Here's how the part is built. I have some questions about the finished solid (model axes, mm). Face numbers are marked on the shaded views. A direction names the side the tool comes from. Round coordinates to 2 decimals unless told otherwise and drop trailing zeros. Loops run counter-clockwise (first coordinate to the right, second up) from the corner with the lowest first, then second, coordinate; pieces in that order, holes last. Notation, with made-up numbers: (41.25, 33) -> (55.25, 33) arc R3 ccw to (55.25, 37) -> close; hole circle Ø5 at (38.5, 23). An arc over 180 degrees is marked (long way). One line per item, written item: value. Start each with the question number.
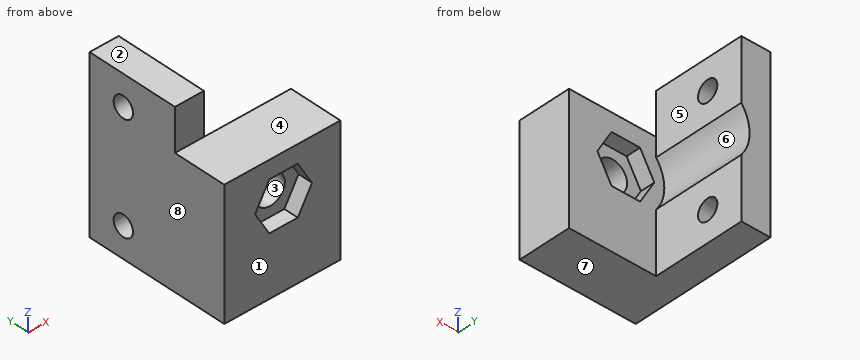
```python
from build123d import *

# Parameters (mm, degrees)
SKETCH1_W           = 18
SKETCH1_H           = 35
SKETCH1_R           = 3.05
BOSS_EXTRUDE1_DEPTH = 11
SKETCH1_3_W         = 6
SKETCH1_3_H         = 35
BOSS_EXTRUDE2_DEPTH = 30
SKETCH2_R           = 7.949273458
CUT_EXTRUDE1_DEPTH  = 19
CUT_EXTRUDE3_DEPTH  = 3
CUT_EXTRUDE4_DEPTH  = 3
SKETCH7_R           = 2.15
CUT_EXTRUDE6_DEPTH  = 10
SKETCH8_W           = 24
SKETCH8_H           = 8.700587772
CUT_EXTRUDE7_DEPTH  = 11


with BuildPart() as part:
    # Sketch1 → Boss-Extrude1 (new body)
    with BuildSketch(Plane(origin=(0, 0, 0), x_dir=(1, 0, 0), z_dir=(0, 1, 0))):
        with Locations((12, 0)):
            Rectangle(SKETCH1_W, SKETCH1_H)
        with Locations((9.25, 0)):
            Circle(SKETCH1_R, mode=Mode.SUBTRACT)
    extrude(amount=BOSS_EXTRUDE1_DEPTH)

    # Sketch1<3> → Boss-Extrude2 (add)
    with BuildSketch(Plane(origin=(0, 0, 0), x_dir=(1, 0, 0), z_dir=(0, 1, 0))):
        Rectangle(SKETCH1_3_W, SKETCH1_3_H)
    extrude(amount=BOSS_EXTRUDE2_DEPTH)

    # Sketch2 → Cut-Extrude1 (cut)
    with BuildSketch(Plane(origin=(0, 30, 0), x_dir=(1, 0, 0), z_dir=(0, 1, 0))):
        with Locations((9.25, 0)):
            Circle(SKETCH2_R)
    extrude(amount=-CUT_EXTRUDE1_DEPTH, mode=Mode.SUBTRACT)

    # Sketch4 → Cut-Extrude3 (cut)
    with BuildSketch(Plane(origin=(0, 11, 0), x_dir=(1, 0, 0), z_dir=(0, 1, 0))):
        Polygon((15.138972746, 0), (12.194486373, 5.1), (6.305513627, 5.1), (3.361027254, 0), (6.305513627, -5.1), (12.194486373, -5.1), align=None)
    extrude(amount=-CUT_EXTRUDE3_DEPTH, mode=Mode.SUBTRACT)

    # Sketch5 → Cut-Extrude4 (cut)
    with BuildSketch(Plane.XZ):
        Polygon((3.361027254, 0), (6.305513627, -5.1), (12.194486373, -5.1), (15.138972746, 0), (12.194486373, 5.1), (6.305513627, 5.1), align=None)
    extrude(amount=-CUT_EXTRUDE4_DEPTH, mode=Mode.SUBTRACT)

    # Sketch7 → Cut-Extrude6 (cut)
    with BuildSketch(Plane(origin=(3, 0, 0), x_dir=(0, 0, -1), z_dir=(1, 0, 0))):
        with Locations((-11.206035856, 22.5)):
            Circle(SKETCH7_R)
        with Locations((11.206035856, 22.5)):
            Circle(SKETCH7_R)
    extrude(amount=-CUT_EXTRUDE6_DEPTH, mode=Mode.SUBTRACT)

    # Sketch8 → Cut-Extrude7 (cut)
    with BuildSketch(Plane.XZ):
        with Locations((9, 13.149706114)):
            Rectangle(SKETCH8_W, SKETCH8_H)
    extrude(amount=-CUT_EXTRUDE7_DEPTH, mode=Mode.SUBTRACT)


solid = part.part
```
Q1. Will these pins go through, and if not, where does the flat tip stop? P1, Ø3.5, axis at y = 22.5, z = -11.21, coming from the +X side; P2, Ø4, axis at y = 17, z = -8, coming from the +X side; P3, Ø2.5, axis at x = 8, y = 2, coming from the +Z side; P4, Ø3, axis at x = 0, z = 12.5, coming from the -Y side.
Q2. I want a section at D-D on z = 6.5. Please give me the cut outline in (x, y), plus the area to 3 significant figures.
Q3. Which directions (+Z, -Z, +X, -X, +Y, -Y) give clear straight access to the entire face, cutting with the end or side of a thin tool? Please do the marked faces 4, 5, 6, 7 and 8.
Q4. I want a section at C-C on y = 22.5. Please give me the cut outline in (x, z), plus the area to 3 significant figures.
Q5. If I drill on line 1 along Z through (x, y) = (9.25, 6.15); line 2 along X through (y, z) = (26, -16); line 3 along Y through (x, z) = (15.75, -12), over which ranges is the centre line in solid material (lowest first)?
Q6. I want a section at B-B on y = 10. Please give me the cut outline in (x, z).
Q7. I want a section at A-A on x = 9.25. Please give me the cut outline in (y, z), plus the area to 3 significant figures.
Q8. If we mould it in two halves opening along Z, with no side actions, what happens to the marked faces 1, 2 and 3? For each: released by +Z, released by -Z, zero draft, split by the parting line, or undercut.
Answers below:
1. P1: passes through
1. P2: stops at x = 3
1. P3: stops at z = 8.8
1. P4: stops at y = 11
2. outline: (-3, 0) -> (21, 0) -> (21, 11) -> (3, 11) -> (3, 30) -> (-3, 30) -> close
2. area: 378 mm^2
3. face 4: +Z, +X, -X, -Y
3. face 5: +Z, -Z, +X, +Y
3. face 6: +X, +Y
3. face 7: -Z, +X, -X, +Y, -Y
3. face 8: +Z, -Z, -X, +Y, -Y
4. outline: (-3, -17.5) -> (3, -17.5) -> (3, -13.36) -> (-3, -13.36) -> close; (-3, -9.06) -> (3, -9.06) -> (3, -4.91) arc R7.95 cw to (3, 4.91) -> (3, 9.06) -> (-3, 9.06) -> close; (-3, 13.36) -> (3, 13.36) -> (3, 17.5) -> (-3, 17.5) -> close
4. area: 147 mm^2
5. line 1: z = -17.5 to -3.05, 3.05 to 8.8
5. line 2: x = -3 to 3
5. line 3: y = 0 to 11
6. outline: (-3, -17.5) -> (21, -17.5) -> (21, 8.8) -> (-3, 8.8) -> close; hole (3.36, 0) -> (6.31, -5.1) -> (12.19, -5.1) -> (15.14, 0) -> (12.19, 5.1) -> (6.31, 5.1) -> close
7. outline: (0, -17.5) -> (11, -17.5) -> (11, -5.1) -> (8, -5.1) -> (8, -3.05) -> (3, -3.05) -> (3, -5.1) -> (0, -5.1) -> close; (0, 5.1) -> (3, 5.1) -> (3, 3.05) -> (8, 3.05) -> (8, 5.1) -> (11, 5.1) -> (11, 8.8) -> (0, 8.8) -> close
7. area: 198 mm^2
8. face 1: zero draft
8. face 2: released by +Z
8. face 3: undercut
